```python
from build123d import *
from OCP.BRepFilletAPI import BRepFilletAPI_MakeChamfer

# Parameters (mm, degrees)
SKETCH1_R           = 37.5
BOSS_EXTRUDE1_DEPTH = 263.66978
SKETCH2_R           = 14.780743644
CUT_EXTRUDE1_DEPTH  = 269.950279578
CHAMFER1_SIZE       = 2.120968
CHAMFER1_SIZE2      = 1.224542


with BuildPart() as part:
    # Sketch1 → Boss-Extrude1 (new body)
    with BuildSketch(Plane(origin=(0, 0, 0), x_dir=(1, 0, 0), z_dir=(0, 1, 0))):
        with Locations(Location((0, 0, 0), (0, 0, 270))):
            Circle(SKETCH1_R)
    extrude(amount=BOSS_EXTRUDE1_DEPTH)

    # Sketch2 → Cut-Extrude1 (cut, through all)
    with BuildSketch(Plane(origin=(0, 0, 0), x_dir=(1, 0, 0), z_dir=(0, 1, 0))):
        with Locations(Location((0, 0, 0), (0, 0, 270))):
            Circle(SKETCH2_R)
    extrude(amount=CUT_EXTRUDE1_DEPTH, mode=Mode.SUBTRACT)

    # Chamfer1: one chamfer whose edges measure the first distance from different faces: ONE call of the kernel's chamfer builder (chamfer() names one face for all edges)
    chamfer1_edges_1 = [part.edges().sort_by_distance(p)[0] for p in [
        (0, 0, -37.5),
    ]]
    chamfer1_side_1 = [part.faces().sort_by_distance(p)[0] for p in [
        (0, 131.83489, -37.5),
    ]]
    chamfer1_edges_2 = [part.edges().sort_by_distance(p)[0] for p in [
        (0, 263.66978, -37.5),
    ]]
    chamfer1_side_2 = [part.faces().sort_by_distance(p)[0] for p in [
        (0, 263.66978, -36.439339828),
    ]]
    chamfer1 = BRepFilletAPI_MakeChamfer(part.part.solid().wrapped)
    for e in chamfer1_edges_1:
        chamfer1.Add(CHAMFER1_SIZE, CHAMFER1_SIZE2, e.wrapped, chamfer1_side_1[0].wrapped)  # the first distance lies on this face
    for e in chamfer1_edges_2:
        chamfer1.Add(CHAMFER1_SIZE, CHAMFER1_SIZE2, e.wrapped, chamfer1_side_2[0].wrapped)  # the first distance lies on this face
    add(Compound.cast(chamfer1.Shape()), mode=Mode.REPLACE)


solid = part.part
```
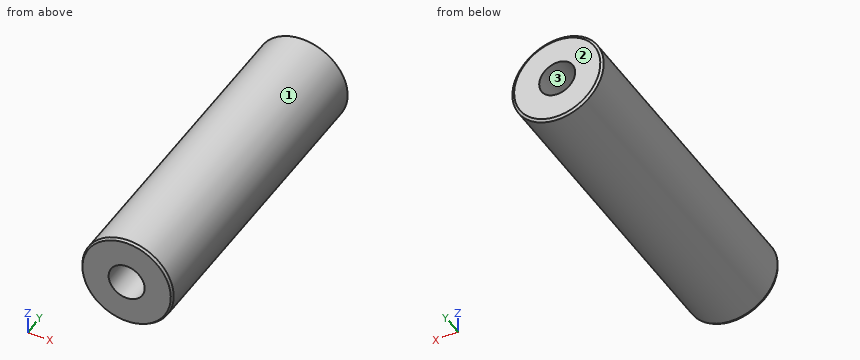
Design review of the part built by this model. Coordinates are the model's own, in mm. Face numbers are marked on the shaded views. Give positions to 0.01 mm unless a question says otherwise; leave off trailing zeros. Write each loop counter-clockwise with the first axis right and the second up, starting at its lowest first coordinate (ties: lowest second). Pieces come first, ordered by that corner, then holes.
(1) Add section C-C (y = 183.5). Give the boundary of the cut face in (x, z), and give its area (3 significant figures).
Checked values:
outline: circle Ø75 at (0, 0); hole circle Ø29.56 at (0, 0)
area: 3,730 mm2
(2) Add section B-B (z = 0). Give the boundary of the cut face in (x, y).
Checked values:
outline: (-37.5, 2.12) - (-36.28, 0) - (-14.78, 0) - (-14.78, 263.67) - (-35.38, 263.67) - (-37.5, 262.45) - close; (14.78, 0) - (36.28, 0) - (37.5, 2.12) - (37.5, 262.45) - (35.38, 263.67) - (14.78, 263.67) - close
(3) Clearance check with flat-ended pins moving along their axes: pin 1 Ø3 at (y, z) = (107, -12) entering from -X; pin 2 Ø1 at (y, z) = (200.5, 16.5) entering from -X; pin 3 Ø5 at (y, z) = (224.5, -14) entering from -X. State where each tip first meets the part, or that it passes through.
Checked values:
pin 1: stops at x = -36
pin 2: stops at x = -33.92
pin 3: stops at x = -35.69
(4) Wall thickness on line 1 along X through (y, z) = (195, 0); line 2 along Z through (x, y) = (9.5, 200); line 3 along X through (y, z) = (68.5, -12.5): over which ranges is each line inside the solid? List them lowest first.
Checked values:
line 1: x = -37.5 to -14.78, 14.78 to 37.5
line 2: z = -36.28 to -11.32, 11.32 to 36.28
line 3: x = -35.36 to -7.89, 7.89 to 35.36
(5) Mouldability with a two-part tool opening along Z and no side actions: class the marked faces 1, 2 and 3 as +Z half, -Z half, draft (parallel to the pull), parting line (faces both ways), or undercut.
Checked values:
face 1: parting line
face 2: draft
face 3: undercut
(6) Add section A-A (x = 0). Give the boundary of the cut face in (y, z), and give its area (3 significant figures).
Checked values:
outline: (0, -36.28) - (2.12, -37.5) - (262.45, -37.5) - (263.67, -35.38) - (263.67, -14.78) - (0, -14.78) - close; (0, 14.78) - (263.67, 14.78) - (263.67, 35.38) - (262.45, 37.5) - (2.12, 37.5) - (0, 36.28) - close
area: 12,000 mm2
